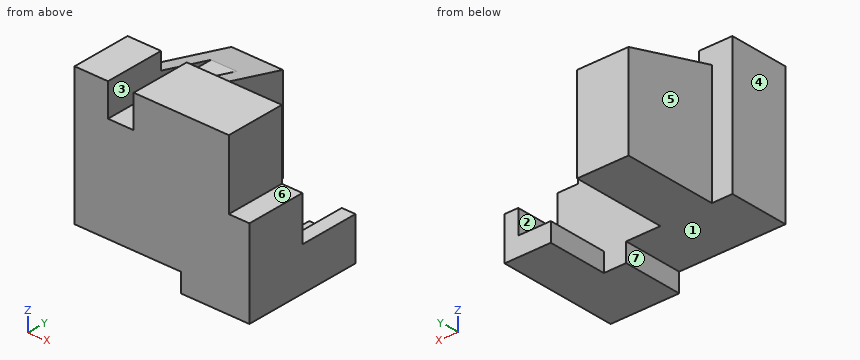
from build123d import *

# Parameters (mm, degrees)
EXTRUDE_1_DEPTH     = 80
EXTRUDE_START       = -12
EXTRUDE_2_DEPTH     = 30
SKETCH_3_W          = 15
SKETCH_3_H          = 19
CUT_EXTRUDE_1_DEPTH = 129.549601322
SKETCH_4_W          = 12
SKETCH_4_H          = 26
SKETCH_4_W_2        = 13
SKETCH_4_H_2        = 11
EXTRUDE_3_DEPTH     = 35
EXTRUDE_4_DEPTH     = 35
SKETCH_5_W          = 4
SKETCH_5_H          = 14
CUT_EXTRUDE_2_DEPTH = 35
EXTRUDE_5_DEPTH     = 40


with BuildPart() as part:
    # Эскиз1 → Бобышка-Вытянуть1 (new body)
    with BuildSketch(Plane.XY):
        Polygon((-45, -17.5), (30, -17.5), (45, 17.5), (-45, 17.5), align=None)
    extrude(amount=EXTRUDE_1_DEPTH)

    # Эскиз2 → Бобышка-Вытянуть2 (add)
    with BuildSketch(Plane.ZY.offset(45).offset(EXTRUDE_START)):
        Polygon((0, 17.5), (0, 72.5), (55, 72.5), (70, 17.5), align=None)
    extrude(amount=-EXTRUDE_2_DEPTH)

    # Эскиз3 → Вырез-Вытянуть1 (cut, through all)
    with BuildSketch(Plane(origin=(0, 72.5, 0), x_dir=(1, 0, 0), z_dir=(0, 1, 0))):
        with Locations((-18, -70.5)):
            Rectangle(SKETCH_3_W, SKETCH_3_H)
    extrude(amount=-CUT_EXTRUDE_1_DEPTH, mode=Mode.SUBTRACT)

    # Эскиз4 → Бобышка-Вытянуть3 (add)
    with BuildSketch(Plane(origin=(0, 17.5, 0), x_dir=(1, 0, 0), z_dir=(0, 1, 0))):
        Polygon((17, 0), (17, -40), (45, -40), (45, -14), (45, 0), (30, 0), align=None)
        with Locations((51, -27)):
            Rectangle(SKETCH_4_W, SKETCH_4_H)
        Polygon((45, 0), (45, -14), (57, -14), (57, 11), (30, 11), (30, 0), align=None)
        with Locations((23.5, 5.5)):
            Rectangle(SKETCH_4_W_2, SKETCH_4_H_2)
    extrude(amount=-EXTRUDE_3_DEPTH)

    # Эскиз4<3> → Бобышка-Вытянуть4 (add)
    with BuildSketch(Plane(origin=(0, 17.5, 0), x_dir=(1, 0, 0), z_dir=(0, 1, 0))):
        Polygon((45, 0), (45, -14), (57, -14), (57, 11), (30, 11), (30, 0), align=None)
    extrude(amount=EXTRUDE_4_DEPTH)

    # Эскиз5 → Вырез-Вытянуть2 (cut)
    with BuildSketch(Plane(origin=(0, 52.5, 0), x_dir=(1, 0, 0), z_dir=(0, 1, 0))):
        with Locations((47, -7)):
            Rectangle(SKETCH_5_W, SKETCH_5_H)
    extrude(amount=-CUT_EXTRUDE_2_DEPTH, mode=Mode.SUBTRACT)

    # Эскиз6 → Бобышка-Вытянуть5 (add)
    with BuildSketch(Plane.XY.offset(80)):
        Polygon((30, -17.5), (45, 17.5), (45, -17.5), align=None)
    extrude(amount=-EXTRUDE_5_DEPTH)


solid = part.part
The model under review builds one solid part; all positions refer to its coordinate system, in mm. Face numbers are marked on the shaded views. A direction names the side the tool comes from. Round coordinates to 2 decimals unless told otherwise and drop trailing zeros. Order: outer loops, then holes, each group sorted by start corner. A loop starts at its lowest first (then second) coordinate and runs counter-clockwise, first axis right, second up. Notation, with made-up numbers: (-19, -2.75) - (6, -2.75) arc R35 cw to (6, 31.25) - close; hole circle Ø1 at (69.25, 43.25). An arc over 180 degrees is marked (long way). Use one line per item in the form item = value.
Q1. Mouldability with a two-part tool opening along X and no side actions: class the marked faces 1, 2, 3 and 4 as pulls with the +X half, pulls with the -X half, needs draft (parallel to the pull), parting line crosses it, or undercut.
Response values:
face_1 = needs draft
face_2 = undercut
face_3 = undercut
face_4 = pulls with the -X half
Q2. Clearance check with flat-ended pins moving along their axes: P1, Ø9.5, axis at x = 49, y = -4.5, coming from the +Z side; P2, Ø5.5, axis at y = 27.5, z = 69, coming from the +X side; P3, Ø5.5, axis at y = 3.5, z = -5.5, coming from the -X side; P4, Ø21, axis at x = 37, y = 38.5, coming from the +Z side. State where each tip first meets the part, or that it passes through.
Response values:
P1 = 80
P2 = -3
P3 = 17
P4 = 0
Q3. Add section C-C on y = -1.5. Give the boundary of the cut face in (x, z).
Response values:
outline = (-45, 0) - (17, 0) - (17, -11) - (57, -11) - (57, 40) - (45, 40) - (45, 80) - (-10.5, 80) - (-10.5, 61) - (-25.5, 61) - (-25.5, 80) - (-45, 80) - close
Q4. Add section A-A on z = 9. Give the boundary of the cut face in (x, y), then the cut area to 3 significant figures.
Response values:
outline = (-45, -17.5) - (57, -17.5) - (57, 52.5) - (49, 52.5) - (49, 17.5) - (-3, 17.5) - (-3, 72.5) - (-33, 72.5) - (-33, 17.5) - (-45, 17.5) - close
area = 5,500 mm^2
Q5. Add section B-B on y = 47. Give the boundary of the cut face in (x, z).
Response values:
outline = (-33, 0) - (-3, 0) - (-3, 61.95) - (-10.5, 61.95) - (-10.5, 61) - (-25.5, 61) - (-25.5, 61.95) - (-33, 61.95) - close; (30, -11) - (57, -11) - (57, 14) - (49, 14) - (49, 0) - (30, 0) - close
Q6. Tool access review of the marked faces 5, 6 and 7: name each direction out of +Z, -Z, +X, -X, +Y, -Y from which nothing blocks a thin tool from reaching the whole face with its end or side.
Response values:
face_5 = +Z, -Z, -X, +Y
face_6 = +Z, +X, +Y, -Y
face_7 = -Z, -X, +Y, -Y
Q7. Add section D-D on x = 36. Give the boundary of the cut face in (y, z), then the cut area to 3 significant figures.
Response values:
outline = (-17.5, -11) - (52.5, -11) - (52.5, 0) - (17.5, 0) - (17.5, 80) - (-17.5, 80) - close
area = 3,570 mm^2
Q8. To check wall thickness, follow line 1 (X direction, y = -7.5, z = 62); line 2 (X direction, y = 52, z = -3); line 3 (Y direction, x = 17, z = 8). State the ranges of each line that lie inside material, in increasing order.
Response values:
line_1 = -45 to -25.5, -10.5 to 45
line_2 = 30 to 57
line_3 = -17.5 to 17.5
